```python
from build123d import *

# Parameters (mm, degrees)
BOSS_EXTRUDE1_DEPTH = 3
SKETCH3_R           = 4.5
CUT_EXTRUDE1_DEPTH  = 7


with BuildPart() as part:
    # Sketch2 → Boss-Extrude1 (new body, symmetric)
    with BuildSketch(Plane(origin=(0, 0, 0), x_dir=(1, 0, 0), z_dir=(0, 1, 0))):
        Polygon((-4.5, 7.794228634), (-9, 0), (-4.5, -7.794228634), (4.5, -7.794228634), (9, 0), (4.5, 7.794228634), align=None)
    extrude(amount=BOSS_EXTRUDE1_DEPTH, both=True)

    # Sketch3 → Cut-Extrude1 (cut, through all)
    with BuildSketch(Plane(origin=(0, 3, 0), x_dir=(1, 0, 0), z_dir=(0, 1, 0))):
        with Locations(Location((0, 0, 0), (0, 0, 270))):  # turned: the seam where the file's is
            Circle(SKETCH3_R)
    extrude(amount=-CUT_EXTRUDE1_DEPTH, mode=Mode.SUBTRACT)

    # Sketch10 → Cut-Revolve1 (revolve, cut)
    with BuildSketch(Plane.XY, mode=Mode.PRIVATE) as cut_revolve1_sk:
        Polygon((-9, 3), (-9, 2.191556781), (-7.599735269, 3), align=None)
    cut_revolve1 = revolve(cut_revolve1_sk.sketch.rotate(Axis((0, 0, 0), (0, 1, 0)), 90), axis=Axis((0, 0, 0), (0, 1, 0)), mode=Mode.SUBTRACT)  # turned: the seam where the file's is

    # Mirror1: Cut-Revolve1 across plane
    add(cut_revolve1.mirror(Plane.ZX), mode=Mode.SUBTRACT)


solid = part.part
```
Could you check a few things on this model? Use its own coordinates, in mm. Coordinates: 2 decimals unless noted, no trailing zeros. Order: outer loops, then holes, each group sorted by start corner. A loop starts at its lowest first (then second) coordinate and runs counter-clockwise, first axis right, second up. Notation, with made-up numbers: M 31,-6.75 L 84,-6.75 A31 cw 84,26.25 Z; hole C -27,8 d3. An arc over 180 degrees is marked long. Use a Markdown table: item, result. Add a question column.
Q1. If I drill on L1, parallel to Z at x = 3.75, y = 0.75; L2, parallel to Z at x = 1.25, y = 1.95; L3, parallel to X at y = -1, z = 2, over which ranges is the centre line in solid material (lowest first)?
Q2. I want a section at C-C on y = -2.5. List the corners of the cut face in (x, z) for me.
Q3. I'm going to push a flat-ended pin straight in: pin 1 (8 mm diameter, centred on x = 0, z = 0, fed in from -Y). Where does the tip first touch, or does it pass through?
Q4. I want a section at A-A on y = 0.2. List the corners of the cut face in (x, z) for me, then the cut area to 3 significant figures.
Q5. We'd pull the mould along Z, two halves only. Please class faces 1 (the cylindrical face through (1.352, 0.042, 4.292)), 2 (the flat face through (0, 0, 7.794)), 3 (the flat face through (3.3, -3, 3.3)): pulls with the +Z half, pulls with the -Z half, needs draft (parallel to the pull), parting line crosses it, or undercut.
Q6. I want a section at B-B on x = 0. List the corners of the cut face in (y, z) for me.
Checked values:
| question | item | result |
|---|---|---|
| 1 | L1 | -7.79 to -2.49, 2.49 to 7.79 |
| 1 | L2 | -7.79 to -4.32, 4.32 to 7.79 |
| 1 | L3 | -7.85 to -4.03, 4.03 to 7.85 |
| 2 | outline | M -8.4,-1.04 L -5.1,-6.76 A8.47 ccw -3.3,-7.79 L 3.3,-7.79 A8.47 ccw 5.1,-6.76 L 8.4,-1.04 A8.47 ccw 8.4,1.04 L 5.1,6.76 A8.47 ccw 3.3,7.79 L -3.3,7.79 A8.47 ccw -5.1,6.76 L -8.4,1.04 A8.47 ccw Z; hole C 0,0 d9 |
| 3 | pin 1 | through |
| 4 | outline | M -9,0 L -4.5,-7.79 L 4.5,-7.79 L 9,0 L 4.5,7.79 L -4.5,7.79 Z; hole C 0,0 d9 |
| 4 | area | 147 mm² |
| 5 | face 1 | undercut |
| 5 | face 2 | pulls with the +Z half |
| 5 | face 3 | needs draft |
| 6 | outline | M -3,-7.6 L -2.89,-7.79 L 2.89,-7.79 L 3,-7.6 L 3,-4.5 L -3,-4.5 Z; M -3,4.5 L 3,4.5 L 3,7.6 L 2.89,7.79 L -2.89,7.79 L -3,7.6 Z |
